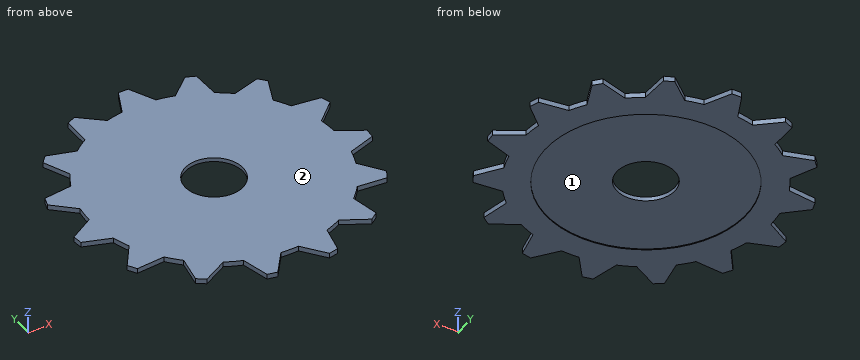
```python
from build123d import *

# Parameters (mm, degrees)
SKETCH1_R           = 31.75
BOSS_EXTRUDE1_DEPTH = 1.27
BOSS_EXTRUDE2_DEPTH = 1.27
SKETCH3_R           = 7.366
CUT_EXTRUDE1_DEPTH  = 10
CIRPATTERN1_COUNT   = 15
SKETCH4_R           = 25.4
CUT_EXTRUDE2_DEPTH  = 0.254


with BuildPart() as part:
    # Sketch1 → Boss-Extrude1 (new body)
    with BuildSketch(Plane.XY):
        Circle(SKETCH1_R)
    extrude(amount=BOSS_EXTRUDE1_DEPTH)

    # Sketch2 → Boss-Extrude2 (add)
    with BuildSketch(Plane.XY.offset(1.27)):
        with BuildLine():
            Line((-1.27, 38.1), (1.27, 38.1))
            Line((1.27, 38.1), (4.372096767, 31.447532015))
            ThreePointArc((4.372096767, 31.447532015), (0, 31.75), (-4.372096767, 31.447532015))
            Line((-4.372096767, 31.447532015), (-1.27, 38.1))
        make_face()
    boss_extrude2 = extrude(amount=-BOSS_EXTRUDE2_DEPTH)

    # Sketch3 → Cut-Extrude1 (cut)
    with BuildSketch(Plane(origin=(0, 0, 0), x_dir=(-1, 0, 0), z_dir=(0, 0, -1))):
        Circle(SKETCH3_R)
    extrude(amount=-CUT_EXTRUDE1_DEPTH, mode=Mode.SUBTRACT)

    # CirPattern1: Boss-Extrude2 ×15 about axis
    cirpattern1_axis = Axis((0, 0, 0), (0, 0, 1))
    for i in range(1, CIRPATTERN1_COUNT):
        add(boss_extrude2.rotate(cirpattern1_axis, i * 360 / CIRPATTERN1_COUNT))

    # Sketch4 → Cut-Extrude2 (cut)
    with BuildSketch(Plane(origin=(0, 0, 0), x_dir=(-1, 0, 0), z_dir=(0, 0, -1))):
        Circle(SKETCH4_R)
    extrude(amount=-CUT_EXTRUDE2_DEPTH, mode=Mode.SUBTRACT)


solid = part.part
```
Model file for the job. Use its own axes, mm. Face numbers are marked on the shaded views. A direction names the side the tool comes from. Coordinates: 2 decimals unless noted, no trailing zeros. Order: outer loops, then holes, each group sorted by start corner. A loop starts at its lowest first (then second) coordinate and runs counter-clockwise, first axis right, second up. Notation, with made-up numbers: (66.25, 23) - (70.25, 23) arc R27 ccw to (70.25, 50) - close; hole circle Ø2 at (50.5, 45). An arc over 180 degrees is marked (long way). Return JSON: item names as keys, results as strings. Group by question number.
1) Probe line 1 (Y direction, x = 0, z = 1.05); line 2 (X direction, y = 35, z = 0.25); line 3 (Y direction, x = -33, z = 0.9). List the from-to ranges inside material, lowest first. Write a range as from..to.
2) Tool access for the marked faces 1 and 2: list every direction of +Z, -Z, +X, -X, +Y, -Y with a clear straight run to the whole face (end or side of a thin tool).
3) Saw through at B-B, the plane y = 0. Write the cut outline in (x, z), plus the area to 3 significant figures.
4) Saw through at A-A, the plane x = 0. Write the cut outline in (y, z).
5) Saw through at D-D, the plane y = -10. Write the cut outline in (x, z), plus the area to 3 significant figures.
6) Saw through at C-C, the plane x = 13. Write the cut outline in (y, z), plus the area to 3 significant figures.
7) Flat gauge pin, fed straight in: P1, Ø23.5, axis at x = 0, y = 0, coming from the -Z side. Where does the tip first touch, or does it go through?
Values found:
{
 "1": {"line 1": "y = -31.75..-7.37, 7.37..38.1", "line 2": "x = -15.06..-13.97, -2.72..2.72, 13.97..15.06", "line 3": "y = -19.04..-17.05, -6.88..0.3, 7.18..13.33"},
 "2": {"face 1": "-Z", "face 2": "+Z, +X, -X, +Y, -Y"},
 "3": {"outline": "(-33.5, 0) - (-25.4, 0) - (-25.4, 0.25) - (-7.37, 0.25) - (-7.37, 1.27) - (-33.5, 1.27) - close; (7.37, 0.25) - (25.4, 0.25) - (25.4, 0) - (33.5, 0) - (33.5, 1.27) - (7.37, 1.27) - close", "area": "57.2 mm²"},
 "4": {"outline": "(-31.75, 0) - (-25.4, 0) - (-25.4, 0.25) - (-7.37, 0.25) - (-7.37, 1.27) - (-31.75, 1.27) - close; (7.37, 0.25) - (25.4, 0.25) - (25.4, 0) - (38.1, 0) - (38.1, 1.27) - (7.37, 1.27) - close"},
 "5": {"outline": "(-30.13, 0) - (-23.35, 0) - (-23.35, 0.25) - (23.35, 0.25) - (23.35, 0) - (30.13, 0) - (30.13, 1.27) - (-30.13, 1.27) - close", "area": "64.7 mm²"},
 "6": {"outline": "(-28.97, 0) - (-21.82, 0) - (-21.82, 0.25) - (21.82, 0.25) - (21.82, 0) - (34.16, 0) - (34.16, 1.27) - (-28.97, 1.27) - close", "area": "69.1 mm²"},
 "7": {"P1": "stops at z = 0.25"}
}
